The figure shows three views and two pictorial views of one solid part (mm, origin at its lowest corner). Answer the questions. A direction names the side the tool comes from. Give positions to 0.01 mm unless a question says otherwise; leave off trailing zeros. Order: outer loops, then holes, each group sorted by start corner. A loop starts at its lowest first (then second) coordinate and runs counter-clockwise, first axis right, second up. Notation, with made-up numbers: M -21,-34.5 L 37,-34.5 A10 cw 37,-16.5 Z; hole C 65,47.5 d1. An arc over 180 degrees is marked long. One line per item, written item: value.
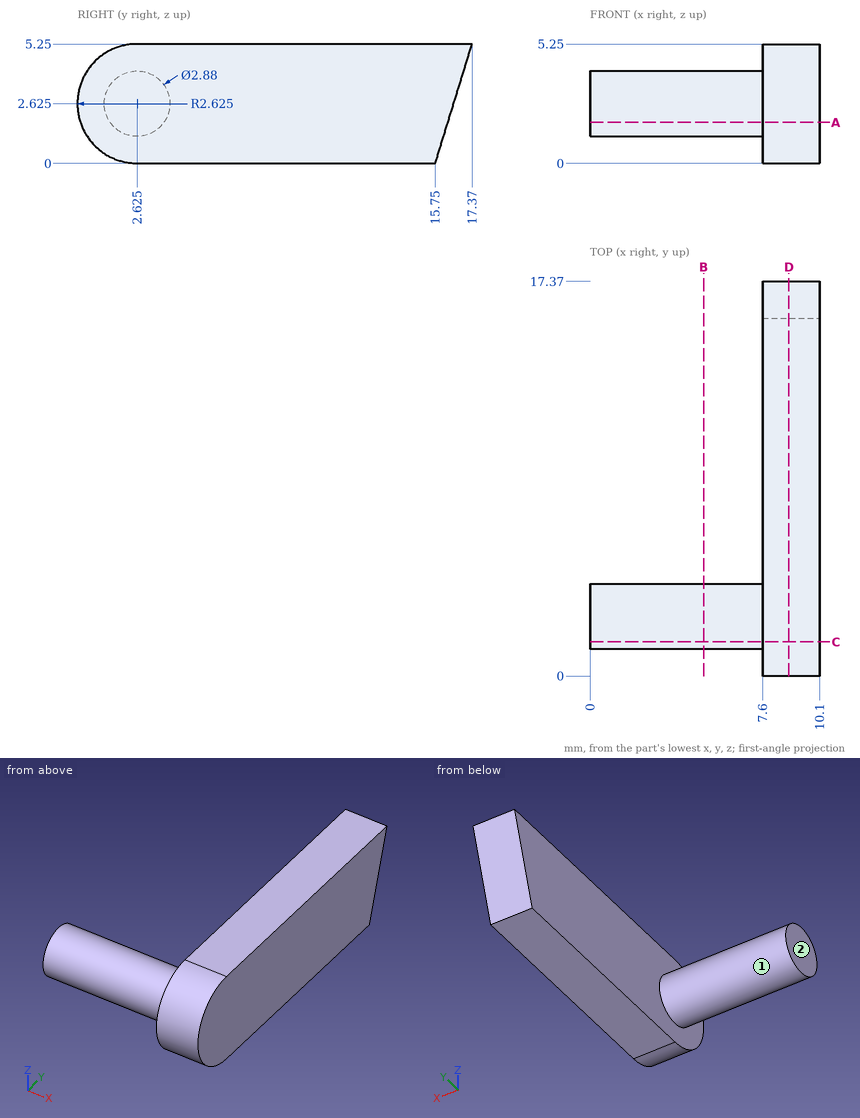
1) Find section A-A, the plane z = 1.8. Write down the section's boundary in (x, y).
Reported:
outline: M 0,1.44 L 7.6,1.44 L 7.6,0.13 L 10.1,0.13 L 10.1,16.31 L 7.6,16.31 L 7.6,3.81 L 0,3.81 Z
2) Which of the six approach directions +Z, -Z, +X, -X, +Y, -Y give full straight-line access (tool end or side, diameter ignored) to the marked faces 1 and 2?
Reported:
face 1: -X
face 2: +Z, -Z, -X, +Y, -Y
3) Find section C-C, the plane y = 1.5. Write down the section's boundary in (x, z), plus the area to 3 significant figures.
Reported:
outline: M 0,1.73 L 7.6,1.73 L 7.6,0.25 L 10.1,0.25 L 10.1,5 L 7.6,5 L 7.6,3.52 L 0,3.52 Z
area: 25.5 mm^2
4) Find section B-B, the plane x = 5. Write down the section's boundary in (y, z) (3 decimals).
Reported:
outline: C 2.625,2.625 d2.88
5) Find section D-D, the plane x = 8.75. Write down the section's boundary in (y, z) (3 decimals).
Reported:
outline: M 2.625,0 L 15.75,0 L 17.37,5.25 L 2.625,5.25 A2.625 ccw Z
6) Each of these flat-tipped pins is pushed along its axis until it touches: pin 1 Ø6 at (x, y) = (4, 13) entering from +Z; pin 2 Ø3 at (x, z) = (5.5, 3.5) entering from -Y (3 decimals); pin 3 Ø2 at (y, z) = (12, 3.5) entering from -X. Where does it stop, or does it pass through?
Reported:
pin 1: passes through
pin 2: stops at y = 1.185
pin 3: stops at x = 7.6
7) Consider probe 1 along X at (y, z) = (8.25, 2.25); probe 2 along Y at (x, z) = (7.75, 4.65); probe 3 along Y at (x, z) = (8.25, 0.6). Determine where each line is inside the solid, lowest interval first.
Reported:
probe 1: x = 7.6 to 10.1
probe 2: y = 0.95 to 17.18
probe 3: y = 0.95 to 15.94
